The drawing under review shows one solid part. Ordinate dimensions are in mm from its lowest x, y, z. A direction names the side the tool comes from. Coordinates: 2 decimals unless noted, no trailing zeros. Order: outer loops, then holes, each group sorted by start corner. A loop starts at its lowest first (then second) coordinate and runs counter-clockwise, first axis right, second up.
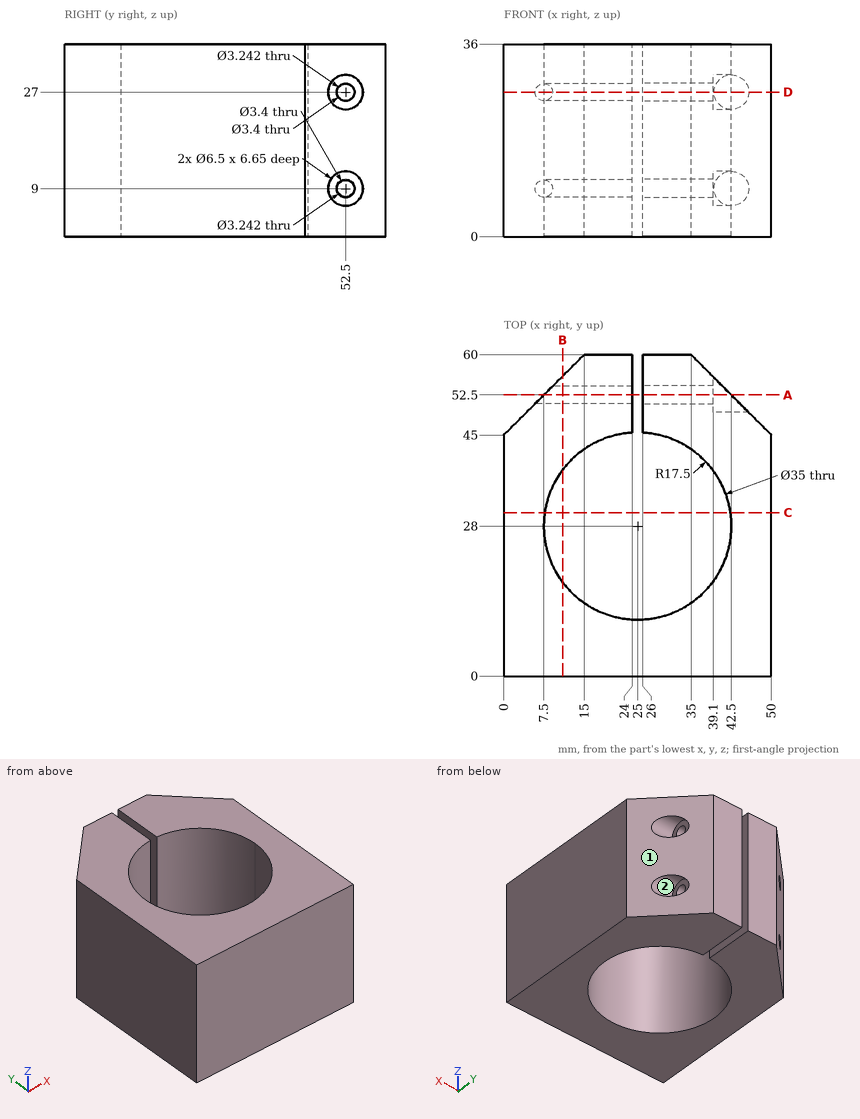
1. Take a section at C-C, the plane y = 30.5. Give the boundary of the cut face in (x, z), plus the area to 3 significant figures.
Answer below:
outline: (0, 0) - (7.68, 0) - (7.68, 36) - (0, 36) - close; (42.32, 0) - (50, 0) - (50, 36) - (42.32, 36) - close
area: 553 mm2
2. Clearance check with flat-ended pins moving along their axes: pin 1 Ø3 at (y, z) = (52, 7.5) entering from +X; pin 2 Ø5 at (y, z) = (53.5, 28) entering from +X; pin 3 Ø11.5 at (y, z) = (56, 11) entering from +X; pin 4 Ø2 at (x, z) = (6.5, 6.5) entering from -Y. State where each tip first meets the part, or that it passes through.
Answer below:
pin 1: stops at x = 39.1
pin 2: stops at x = 42.59
pin 3: stops at x = 44.74
pin 4: stops at y = 0
3. Take a section at D-D, the plane z = 27. Give the boundary of the cut face in (x, y).
Answer below:
outline: (0, 0) - (50, 0) - (50, 45) - (45.75, 49.25) - (39.1, 49.25) - (39.1, 50.8) - (26, 50.8) - (26, 45.47) arc R17.5 cw (long way) to (24, 45.47) - (24, 50.88) - (5.88, 50.88) - (0, 45) - close; (9.12, 54.12) - (24, 54.12) - (24, 60) - (15, 60) - close; (26, 54.2) - (39.1, 54.2) - (39.1, 55.75) - (39.25, 55.75) - (35, 60) - (26, 60) - close
4. Take a section at A-A, the plane y = 52.5. Give the number of separate pieces and of enclosed holes in the cut face, plus the area to 3 significant figures.
Answer below:
separate pieces: 6
enclosed holes: 0
area: 948 mm2
5. Machinability: for the marked faces 1 and 2, which of the approach directions +Z, -Z, +X, -X, +Y, -Y give a long, thin tool a straight path to every point of the face, cutting with its end or side? Answer none if there is none.
Answer below:
face 1: +Z, -Z, +X, +Y
face 2: +X
6. Take a section at B-B, the plane x = 11. Give the boundary of the cut face in (y, z).
Answer below:
outline: (0, 0) - (17.5, 0) - (17.5, 36) - (0, 36) - close; (38.5, 0) - (56, 0) - (56, 36) - (38.5, 36) - close; hole circle Ø3.24 at (52.5, 9); hole circle Ø3.24 at (52.5, 27)
7. To check wall thickness, follow L1, parallel to Z at x = 20, y = 52.5; L2, parallel to X at y = 28.5, z = 23.5; L3, parallel to Z at x = 16, y = 52. State the ranges of each line that lie inside material, in increasing order.
Answer below:
L1: z = 0 to 7.38, 10.62 to 25.38, 28.62 to 36
L2: x = 0 to 7.51, 42.49 to 50
L3: z = 0 to 7.46, 10.54 to 25.46, 28.54 to 36
